Design review of the part built by this model. Coordinates are the model's own, in mm. Face numbers are marked on the shaded views. A direction names the side the tool comes from. Coordinates: 2 decimals unless noted, no trailing zeros. Return JSON: item names as keys, results as strings. Group by question number.
from build123d import *

# Parameters (mm, degrees)
SKETCH1_W           = 36
SKETCH1_H           = 36
BOSS_EXTRUDE1_DEPTH = 186.9
FILLET1_SIZE        = 24
SKETCH2_W           = 14.28
SKETCH2_H           = 23.5
CUT_EXTRUDE1_DEPTH  = 27
SKETCH3_W           = 11.78
SKETCH3_H           = 21
CUT_EXTRUDE2_DEPTH  = 8
SKETCH4_R           = 2
CUT_EXTRUDE3_DEPTH  = 5
BOSS_EXTRUDE2_DEPTH = 4
SKETCH6_W           = 6
SKETCH6_H           = 4
CUT_EXTRUDE4_DEPTH  = 9
SKETCH7_W           = 3
SKETCH7_H           = 3
SKETCH7_W_2         = 12
SKETCH7_H_2         = 12
CUT_EXTRUDE5_DEPTH  = 10
SKETCH8_W           = 9
SKETCH8_H           = 6
CUT_EXTRUDE6_DEPTH  = 2


with BuildPart() as part:
    # Sketch1 → Boss-Extrude1 (new body)
    with BuildSketch(Plane(origin=(0, 0, 0), x_dir=(1, 0, 0), z_dir=(0, 1, 0))):
        with Locations((18, 18)):
            Rectangle(SKETCH1_W, SKETCH1_H)
    extrude(amount=BOSS_EXTRUDE1_DEPTH)

    # Fillet1
    # a fillet whose section is not a circle: 24 mm, written as the material it takes off along each edge
    with BuildSketch(Plane(origin=(36, -60, 0), x_dir=(-1, 0, 0), z_dir=(0, 1, 0))) as fillet1_piece_1:
        with BuildLine():
            Bezier((FILLET1_SIZE, 0), (0, 0), (0, -FILLET1_SIZE), weights=[1, 1.222222222, 1])
            Line((0, -FILLET1_SIZE), (0, 0))
            Line((0, 0), (FILLET1_SIZE, 0))
        make_face()
    extrude(amount=306.9, mode=Mode.SUBTRACT)

    # Sketch2 → Cut-Extrude1 (cut)
    with BuildSketch(Plane.XZ):
        with Locations((7.14, -24.25)):
            Rectangle(SKETCH2_W, SKETCH2_H)
    extrude(amount=-CUT_EXTRUDE1_DEPTH, mode=Mode.SUBTRACT)

    # Sketch3 → Cut-Extrude2 (cut)
    with BuildSketch(Plane.XZ.offset(-27)):
        with Locations((5.89, -25.5)):
            Rectangle(SKETCH3_W, SKETCH3_H)
    extrude(amount=-CUT_EXTRUDE2_DEPTH, mode=Mode.SUBTRACT)

    # Sketch4 → Cut-Extrude3 (cut)
    with BuildSketch(Plane.XZ):
        with Locations(Location((21, -15, 0), (0, 0, 270))):
            Circle(SKETCH4_R)
    extrude(amount=-CUT_EXTRUDE3_DEPTH, mode=Mode.SUBTRACT)

    # Sketch5 → Boss-Extrude2 (add)
    with BuildSketch(Plane.XZ):
        Polygon((18, -28), (22, -28), (22, -24), (28, -24), (28, -28), (32, -28), (32, -32), (18, -32), align=None)
        Polygon((4, -2), (8, -2), (8, -4), (12, -4), (12, -8), (8, -8), (8, -10), (4, -10), align=None)
    extrude(amount=BOSS_EXTRUDE2_DEPTH)

    # Sketch6 → Cut-Extrude4 (cut)
    with BuildSketch(Plane(origin=(0, 0, -36), x_dir=(-1, 0, 0), z_dir=(0, 0, -1))):
        with Locations((-29, 180.9)):
            Rectangle(SKETCH6_W, SKETCH6_H)
        with Locations((-7, 180.9)):
            Rectangle(SKETCH6_W, SKETCH6_H)
        with Locations((-29, 160.9)):
            Rectangle(SKETCH6_W, SKETCH6_H)
    extrude(amount=-CUT_EXTRUDE4_DEPTH, mode=Mode.SUBTRACT)

    # Sketch7 → Cut-Extrude5 (cut)
    with BuildSketch(Plane(origin=(0, 186.9, 0), x_dir=(1, 0, 0), z_dir=(0, 1, 0))):
        with Locations((29, 31.5)):
            Rectangle(SKETCH7_W, SKETCH7_H)
        with Locations((18, 18)):
            Rectangle(SKETCH7_W_2, SKETCH7_H_2)
    extrude(amount=-CUT_EXTRUDE5_DEPTH, mode=Mode.SUBTRACT)

    # Sketch8 → Cut-Extrude6 (cut)
    with BuildSketch(Plane(origin=(0, 186.9, 0), x_dir=(1, 0, 0), z_dir=(0, 1, 0))):
        with Locations((29, 30)):
            Rectangle(SKETCH8_W, SKETCH8_H)
    extrude(amount=-CUT_EXTRUDE6_DEPTH, mode=Mode.SUBTRACT)


solid = part.part
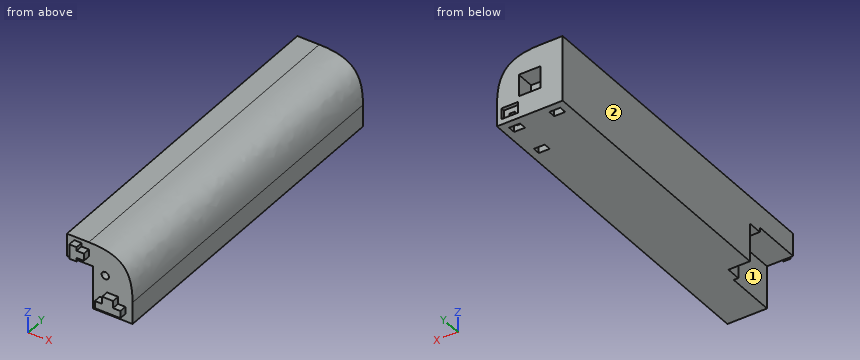
Q1. For the marked faces 1 and 2, list the 3-axis set-ups (+Z, -Z, +X, -X, +Y, -Y) from which the entire face can be reached by the end or side of a thin tool; tool diameter is ignored.
Q2. For P1, Ø5, axis at x = 6.5, z = -32.5, coming from the -Y side; P2, Ø2, axis at x = 22, z = -14, coming from the -Y side; P3, Ø2, axis at x = 24, y = -2, coming from the +Z side, all flat-tipped, find the tip position at first contact; note any pin that passes through.
Q3. Wall thickness on L1, parallel to Y at x = 20.5, z = -2.5; L2, parallel to Y at x = 16, z = -23; L3, parallel to Z at x = 13, y = 62: over which ranges is each line inside the solid? List them lowest first.
Findings below:
{
 "1": {"face 1": "-Z, -X, -Y", "face 2": "+Z, -Z, -X, +Y, -Y"},
 "2": {"P1": "stops at y = 35", "P2": "stops at y = 0", "P3": "stops at z = -24"},
 "3": {"L1": "y = 0 to 186.9", "L2": "y = 0 to 176.9", "L3": "z = -36 to -0.01"}
}
